Input: part model. Units: mm. Frame: model coordinates. A direction names the side the tool comes from. Coordinates: 2 decimals unless noted, no trailing zeros. Loops run counter-clockwise (first coordinate to the right, second up) from the corner with the lowest first, then second, coordinate; pieces in that order, holes last.
Item 1: Section A-A on x = 0. Return loops of the section in (y, z).
Item 2: Section D-D on x = -25.5. Return loops of the section in (y, z).
Item 3: Reachability of faces 4 (the flat face through (-1, -8, 0)), 5 (the cylindrical face through (-7.82, -35.21, 17.6)), 6 (the flat face through (-12.7, 3, 3)) from +Z, -Z, +X, -X, +Y, -Y: full face, straight path, thin tool, end or side. Return the list, or none.
Item 4: Ray query, line 1 along Y through (x, z) = (0, 25); line 2 along X through (y, z) = (24.5, 8.5); line 3 along Z through (x, y) = (19.5, 24.5). Return the intervals inside material, ascending.
Item 5: Section B-B on y = 3. Return loops of the section in (x, z), and give its area (3 significant figures).
Item 6: Pull-direction query (Y, two-part tool) for faces 1 (the flat face through (-21, 32, 5.08)), 2 (the cylindrical face through (-30.235, -23.183, 17.602)), 3 (the flat face through (12.7, 3, 3)); classes: released by +Y, released by -Y, zero draft, split by the parting line, or undercut.
Item 7: Contact query for flat-ended pins moving along their axis: P1, Ø1.5, axis at y = 3.5, z = 2.5, coming from the +X side; P2, Ø1.5, axis at x = -3, z = 1.5, coming from the -Y side; P3, Ø8, axis at x = -0.5, y = -14.5, coming from the +Z side. Output: stop coordinate, or through.
Item 8: Section C-C on y = 26.5. Return loops of the section in (x, z), and give its area (4 significant figures).
```python
from build123d import *

# Parameters (mm, degrees)
F0_R     = 39.37
F1_DEPTH = 5.08
F2_R     = 38.1
F2_R_2   = 36.068
F3_DEPTH = 25.4
F4_W     = 25.4
F4_H     = 5.08
F5_DEPTH = 5.08


with BuildPart() as f1:
    # F0 (on Top) → F1 (new body)
    with BuildSketch(Plane.XY):
        Circle(F0_R)
    extrude(amount=F1_DEPTH)

    # F2 (on face) → F3 (join)
    with BuildSketch(Plane.XY.offset(5.08)):
        Circle(F2_R)
        Circle(F2_R_2, mode=Mode.SUBTRACT)
    extrude(amount=F3_DEPTH)

    # F4 (on face) → F5 (cut)
    with BuildSketch(Plane(origin=(0, 0, 0), x_dir=(1, 0, 0), z_dir=(0, 0, -1))):
        with Locations((0, -2.54)):
            Rectangle(F4_W, F4_H)
    extrude(amount=-F5_DEPTH, mode=Mode.SUBTRACT)


solid = f1.part
```
Results found:
1. outline: (-39.37, 0) - (0, 0) - (0, 5.08) - (-36.07, 5.08) - (-36.07, 30.48) - (-38.1, 30.48) - (-38.1, 5.08) - (-39.37, 5.08) - close; (5.08, 0) - (39.37, 0) - (39.37, 5.08) - (38.1, 5.08) - (38.1, 30.48) - (36.07, 30.48) - (36.07, 5.08) - (5.08, 5.08) - close
2. outline: (-30, 0) - (30, 0) - (30, 5.08) - (28.31, 5.08) - (28.31, 30.48) - (25.51, 30.48) - (25.51, 5.08) - (-25.51, 5.08) - (-25.51, 30.48) - (-28.31, 30.48) - (-28.31, 5.08) - (-30, 5.08) - close
3. face 4: -Z, +X, -X, +Y, -Y
3. face 5: +Z
3. face 6: +Z, -Z
4. line 1: y = -38.1 to -36.07, 36.07 to 38.1
4. line 2: x = -29.18 to -26.47, 26.47 to 29.18
4. line 3: z = 0 to 5.08
5. outline: (-39.26, 0) - (-12.7, 0) - (-12.7, 5.08) - (-35.94, 5.08) - (-35.94, 30.48) - (-37.98, 30.48) - (-37.98, 5.08) - (-39.26, 5.08) - close; (12.7, 0) - (39.26, 0) - (39.26, 5.08) - (37.98, 5.08) - (37.98, 30.48) - (35.94, 30.48) - (35.94, 5.08) - (12.7, 5.08) - close
5. area: 373 mm2
6. face 1: zero draft
6. face 2: split by the parting line
6. face 3: undercut
7. P1: stops at x = 39.27
7. P2: stops at y = -39.31
7. P3: stops at z = 5.08
8. outline: (-29.12, 0) - (29.12, 0) - (29.12, 5.08) - (27.37, 5.08) - (27.37, 30.48) - (24.47, 30.48) - (24.47, 5.08) - (-24.47, 5.08) - (-24.47, 30.48) - (-27.37, 30.48) - (-27.37, 5.08) - (-29.12, 5.08) - close
8. area: 443.5 mm2
